Read the model definition and answer for the solid it produces. Units are mm, in the model's axes. Face numbers are marked on the shaded views. Coordinates: 2 decimals unless noted, no trailing zeros. Loops run counter-clockwise (first coordinate to the right, second up) from the corner with the lowest first, then second, coordinate; pieces in that order, holes last. Notation, with made-up numbers: M 48,42.5 L 104,42.5 A16 ccw 104,68.5 Z; hole C -40,40 d1. An arc over 180 degrees is marked long. One line per item, written item: value. Start each with the question number.
1. Determine the mould class of the marked faces 1, 2 and 3 for opening direction X: +X half, -X half, draft (parallel to the pull), parting line (faces both ways), or undercut.
2. Flat-ended cylindrical pins translate along their axes: pin 1 (3 mm diameter, centred on x = 62, z = -146, fed in from +Y); pin 2 (2 mm diameter, centred on x = 12, z = 139, fed in from -Y); pin 3 (1 mm diameter, centred on x = -59.5, y = 0, fed in from -Z) (3 decimals). Find the tip coordinate at first contact, or state that the pin passes through.
3. The part is cut by section A-A (x = 0). Write down the section's boundary in (y, z) (3 decimals), then the cut area to 3 significant figures.
4. The part is cut by section C-C (z = -171.5). Write down the section's boundary in (x, y) (3 decimals).
5. Consider probe 1 along Z at (x, y) = (-23.5, 73) (3 decimals); probe 2 along Y at (x, z) = (0, -63) (3 decimals); probe 3 along X at (y, z) = (-0.5, -105.5). Determine where each line is inside the solid, lowest interval first.
Autodesk Inventor part; units mm, degrees
ref_plane "YZ Plane" through (0, 0, 0) normal (1, 0, 0) x (0, 1, 0)
ref_plane "XZ Plane" through (0, 0, 0) normal (0, 1, 0) x (-1, 0, 0)
ref_plane "XY Plane" through (0, 0, 0) normal (0, 0, 1) x (1, 0, 0)
sketch "Sketch1" plane through (0, 0, 0) normal (0, 0, 1) x (1, 0, 0)
  circle A0 centre (0, 0) radius 76.2
  dimension "tubeDiameter" = 152.4
extrude "Extrusion1" add sketch "Sketch1" along normal mid plane 438.15
sketch "Sketch2" plane through (0, 0, -219.075) normal (0, 0, -1) x (-1, 0, 0)
  circle A0 centre (0, 0) radius 73.025
  dimension "d6" = 146.05
extrude "Extrusion2" cut sketch "Sketch2" against normal blind 406.4
sketch "Sketch3" plane through (0, 0, 219.075) normal (0, 0, 1) x (1, 0, 0)
  circle A0 centre (0, 0) radius 82.55
  circle A1 centre (0, 0) radius 76.2
  dimension "d9" = 165.1
extrude "Extrusion3" add sketch "Sketch3" against normal blind 25.4
sketch "Sketch4" plane through (0, 0, -219.075) normal (0, 0, -1) x (-1, 0, 0)
  circle A0 centre (0, 0) radius 76.2
  circle A1 centre (0, 0) radius 82.55
extrude "Extrusion4" add sketch "Sketch4" against normal blind 25.4
properties part number "telescopeTube" material "Aluminum 6061"
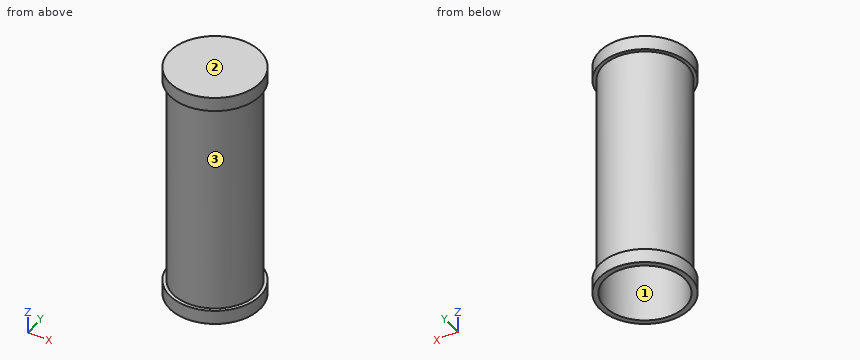
Answer block:
1. face 1: undercut
1. face 2: draft
1. face 3: parting line
2. pin 1: stops at y = 46.33
2. pin 2: stops at y = -75.4
2. pin 3: stops at z = 187.325
3. outline: M -82.55,-219.075 L -73.025,-219.075 L -73.025,187.325 L 73.025,187.325 L 73.025,-219.075 L 82.55,-219.075 L 82.55,-193.675 L 76.2,-193.675 L 76.2,193.675 L 82.55,193.675 L 82.55,219.075 L -82.55,219.075 L -82.55,193.675 L -76.2,193.675 L -76.2,-193.675 L -82.55,-193.675 Z
3. area: 8,060 mm2
4. outline: C 0,0 d152.4; hole C 0,0 d146.05
5. probe 1: z = -219.075 to -193.675, 193.675 to 219.075
5. probe 2: y = -76.2 to -73.025, 73.025 to 76.2
5. probe 3: x = -76.2 to -73.02, 73.02 to 76.2
